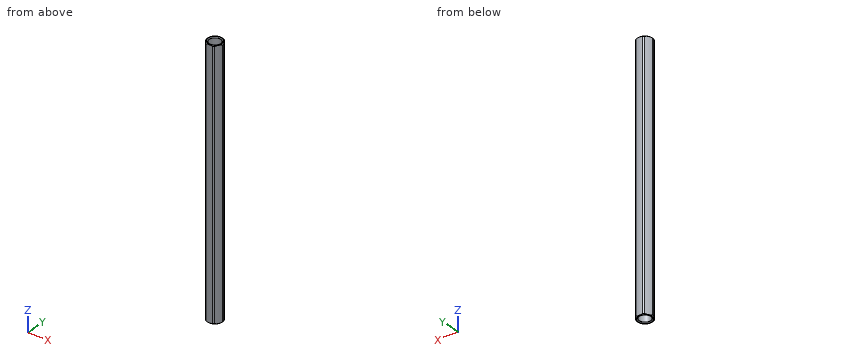
```python
from build123d import *

# Parameters (mm, degrees)
ESBO_O3_R       = 2.9
EXTRUS_O2_DEPTH = 65.85


with BuildPart() as part:
    # Esbo_o3 → Extrus_o2 (new, symmetric)
    with BuildSketch(Plane.XY):
        with BuildLine():
            ThreePointArc((-1.679123513, 3.708327237), (-2.061437209, 3.570513982), (-2.371943836, 3.308327237))
            ThreePointArc((-2.371943836, 3.308327237), (-3.334197805, 1.925), (-4.05106735, 0.4))
            ThreePointArc((-4.05106735, 0.4), (-4.122874417, 0), (-4.05106735, -0.4))
            ThreePointArc((-4.05106735, -0.4), (-3.334197805, -1.925), (-2.371943836, -3.308327237))
            ThreePointArc((-2.371943836, -3.308327237), (-2.061437209, -3.570513982), (-1.679123513, -3.708327237))
            ThreePointArc((-1.679123513, -3.708327237), (0, -3.85), (1.679123513, -3.708327237))
            ThreePointArc((1.679123513, -3.708327237), (2.061437209, -3.570513982), (2.371943836, -3.308327237))
            ThreePointArc((2.371943836, -3.308327237), (3.334197805, -1.925), (4.05106735, -0.4))
            ThreePointArc((4.05106735, -0.4), (4.122874417, 0), (4.05106735, 0.4))
            ThreePointArc((4.05106735, 0.4), (3.334197805, 1.925), (2.371943836, 3.308327237))
            ThreePointArc((2.371943836, 3.308327237), (2.061437209, 3.570513982), (1.679123513, 3.708327237))
            ThreePointArc((1.679123513, 3.708327237), (0, 3.85), (-1.679123513, 3.708327237))
        make_face()
        Circle(ESBO_O3_R, mode=Mode.SUBTRACT)
    extrude(amount=EXTRUS_O2_DEPTH, both=True)

    # Esbo_o5 → Corte-Revolu_o2 (revolve, cut)
    with BuildSketch(Plane(origin=(0, 0, 0), x_dir=(0, 0, -1), z_dir=(1, 0, 0)), mode=Mode.PRIVATE) as corte_revolu_o2_sk:
        Polygon((65.85, 3.73), (65.124884733, 4.455115267), (66.124884733, 4.455115267), (66.124884733, 3.73), align=None)
        Polygon((65.85, 3.4), (65.45, 3), (65.45, 2.769529571), (65.85, 2.769529571), align=None)
        Polygon((-65.85, 3.73), (-66.124884733, 3.73), (-66.124884733, 4.455115267), (-65.124884733, 4.455115267), align=None)
    corte_revolu_o2 = revolve(corte_revolu_o2_sk.sketch.rotate(Axis((0, 0, -65.739939352), (0, 0, 1)), 275.639072873), axis=Axis((0, 0, -65.739939352), (0, 0, 1)), mode=Mode.SUBTRACT)

    # Espelhar1: Corte-Revolu_o2 across plane
    add(corte_revolu_o2.mirror(Plane.XY), mode=Mode.SUBTRACT)


solid = part.part
```
For this review, take the finished solid that the model builds, in its own axes (mm). Round coordinates to 2 decimals unless told otherwise and drop trailing zeros. Write each loop counter-clockwise with the first axis right and the second up, starting at its lowest first coordinate (ties: lowest second). Pieces come first, ordered by that corner, then holes. Notation, with made-up numbers: (77, -27) -> (102, -27) arc R6 cw to (102, -23) -> close; hole circle Ø2 at (12, 78.25). An arc over 180 degrees is marked (long way). Use one line per item in the form item = value.
Q1. Consider section A-A (x = 0). State the section outline as (y, z) points.
Resolved:
outline = (-3.85, -65.73) -> (-3.73, -65.85) -> (-3.4, -65.85) -> (-3, -65.45) -> (-2.9, -65.45) -> (-2.9, 65.45) -> (-3, 65.45) -> (-3.4, 65.85) -> (-3.73, 65.85) -> (-3.85, 65.73) -> close; (2.9, -65.45) -> (3, -65.45) -> (3.4, -65.85) -> (3.73, -65.85) -> (3.85, -65.73) -> (3.85, 65.73) -> (3.73, 65.85) -> (3.4, 65.85) -> (3, 65.45) -> (2.9, 65.45) -> close
Q2. Clearance check with a flat-ended pin moving along its axis: pin 1 Ø1 at (y, z) = (2.5, 34.5) entering from -X. State where the tip first meets the part, or that it passes through.
Resolved:
pin_1 = -3.29
Q3. To check wall thickness, follow probe 1 along Y at (x, z) = (0, 19); probe 2 along X at (y, z) = (0, 28.5); probe 3 along X at (y, z) = (-2, -0.5). State the ranges of each line that lie inside material, in increasing order. Write a range as from..to.
Resolved:
probe_1 = -3.85..-2.9, 2.9..3.85
probe_2 = -4.12..-2.9, 2.9..4.12
probe_3 = -3.29..-2.1, 2.1..3.29
Q4. Consider section B-B (z = 9). State the section outline as (x, y) points.
Resolved:
outline = (-4.05, -0.4) arc R10.02 ccw to (-2.37, -3.31) arc R1.15 ccw to (-1.68, -3.71) arc R10.02 ccw to (1.68, -3.71) arc R1.15 ccw to (2.37, -3.31) arc R10.02 ccw to (4.05, -0.4) arc R1.15 ccw to (4.05, 0.4) arc R10.02 ccw to (2.37, 3.31) arc R1.15 ccw to (1.68, 3.71) arc R10.02 ccw to (-1.68, 3.71) arc R1.15 ccw to (-2.37, 3.31) arc R10.02 ccw to (-4.05, 0.4) arc R1.15 ccw to start; hole circle Ø5.8 at (0, 0)
